Verification items for the finished model (mm, model axes). Face numbers are marked on the shaded views. A direction names the side the tool comes from. Give positions to 0.01 mm unless a question says otherwise; leave off trailing zeros. Order: outer loops, then holes, each group sorted by start corner. A loop starts at its lowest first (then second) coordinate and runs counter-clockwise, first axis right, second up. Notation, with made-up numbers: (24, 20) - (43, 20) arc R21 ccw to (43, 33) - close; hole circle Ø1 at (42, 80.5). An arc over 180 degrees is marked (long way). Answer as a JSON object with one key per item and string values.
```python
from build123d import *

# Parameters (mm, degrees)
SKETCH1_W           = 13
SKETCH1_H           = 8.5
BOSS_EXTRUDE1_DEPTH = 10
BOSS_EXTRUDE2_DEPTH = 6.5


with BuildPart() as part:
    # Sketch1 → Boss-Extrude1 (new body)
    with BuildSketch(Plane(origin=(0, 0, 0), x_dir=(1, 0, 0), z_dir=(0, 1, 0))):
        Rectangle(SKETCH1_W, SKETCH1_H)
    extrude(amount=BOSS_EXTRUDE1_DEPTH)

    # Sketch2 → Boss-Extrude2 (add)
    with BuildSketch(Plane.XY.offset(3.25)):
        Polygon((-5.5, 10), (5.5, 10), (3.5, 11.829740684), align=None)
    extrude(amount=-BOSS_EXTRUDE2_DEPTH)


solid = part.part
```
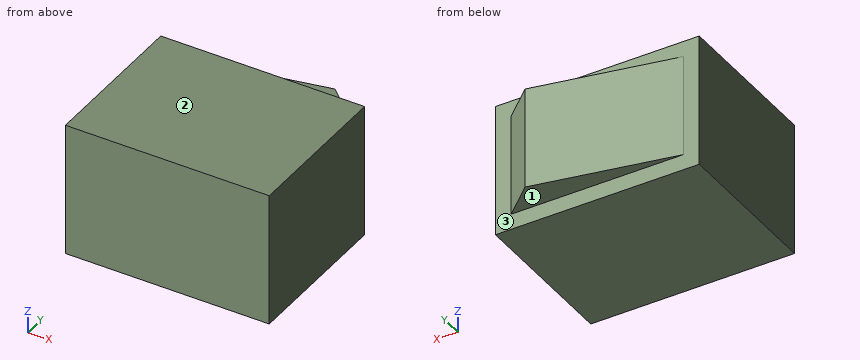
(1) Section check A-A (z = 1.75). Record the cut outline in (x, y).
Computed values:
{"outline": "(-6.5, 0) - (6.5, 0) - (6.5, 10) - (5.5, 10) - (3.5, 11.83) - (-5.5, 10) - (-6.5, 10) - close"}
(2) Section check B-B (x = 0.25). Record the cut outline in (y, z).
Computed values:
{"outline": "(0, -4.25) - (10, -4.25) - (10, -3.25) - (11.17, -3.25) - (11.17, 3.25) - (10, 3.25) - (10, 4.25) - (0, 4.25) - close"}
(3) Access from +Z, -Z, +X, -X, +Y, -Y to the whole of each face (thin tool, end or side, straight path). Record for the marked faces 1, 2 and 3.
Computed values:
{"face 1": "-Z, +X, -X, +Y", "face 2": "+Z, +X, -X, +Y, -Y", "face 3": "+Y"}
(4) Section check C-C (y = 11). Record the cut outline in (x, z), then the cut area to 3 significant figures.
Computed values:
{"outline": "(-0.58, -3.25) - (4.41, -3.25) - (4.41, 3.25) - (-0.58, 3.25) - close", "area": "32.4 mm²"}
(5) Gauge pin test, flat ends, axial feed: pin 1 Ø2.5 at (x, z) = (1.5, 0) entering from +Y; pin 2 Ø1.5 at (x, y) = (-0.5, 11) entering from +Z; pin 3 Ø5 at (x, z) = (-0.5, 1.5) entering from +Y. Record the tip position at first contact, or that the pin passes through.
Computed values:
{"pin 1": "stops at y = 11.68", "pin 2": "stops at z = 3.25", "pin 3": "stops at y = 11.52"}
(6) Material ranges on line 1 along Y through (x, z) = (0, -4); line 2 along Y through (x, z) = (-3.75, 2.5), recorded low to high. Write a range as [from, to].
Computed values:
{"line 1": "y = [0, 10]", "line 2": "y = [0, 10.36]"}
(7) Section check D-D (x = -2.5). Record the cut outline in (y, z).
Computed values:
{"outline": "(0, -4.25) - (10, -4.25) - (10, -3.25) - (10.61, -3.25) - (10.61, 3.25) - (10, 3.25) - (10, 4.25) - (0, 4.25) - close"}
